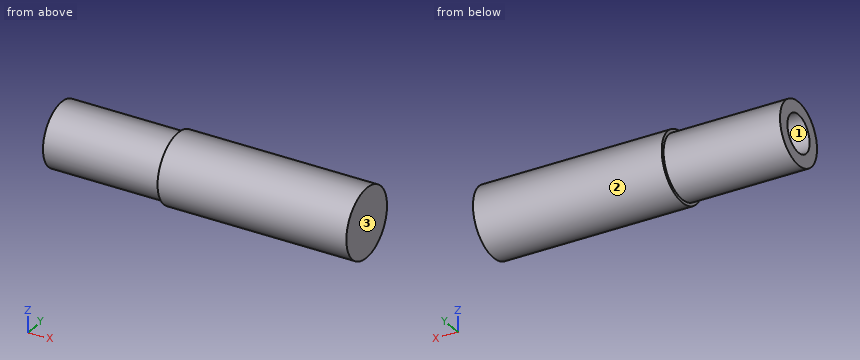
from build123d import *

# Parameters (mm, degrees)
ESQUISSE2_OUTSIDE_W = 23.186
ESQUISSE2_OUTSIDE_H = 23.186
ESQUISSE2_OUTSIDE_R = 5
EXTRUSION1_DEPTH    = 18.5


with BuildPart() as part:
    # Esquisse1 → Révolution1 (revolve)
    with BuildSketch(Plane.XY, mode=Mode.PRIVATE) as r_volution1_sk:
        Polygon((0, 0), (-48.5, 0), (-48.5, -2.5), (-35.5, -2.5), (-35.5, -5.5), (0, -5.5), align=None)
    revolve(r_volution1_sk.sketch.rotate(Axis((-35.5, -5.5, 0), (1, 0, 0)), 180), axis=Axis((-35.5, -5.5, 0), (1, 0, 0)))

    # Esquisse2 outside → Extrusion1 (cut)
    with BuildSketch(Plane.ZY.offset(48.5)):
        with Locations((0, -5.5)):
            Rectangle(ESQUISSE2_OUTSIDE_W, ESQUISSE2_OUTSIDE_H)
        with Locations(Location((0, -5.5, 0), (0, 0, 270))):
            Circle(ESQUISSE2_OUTSIDE_R, mode=Mode.SUBTRACT)
    extrude(amount=-EXTRUSION1_DEPTH, mode=Mode.SUBTRACT)


solid = part.part
Design review of the part built by this model. Coordinates are the model's own, in mm. Face numbers are marked on the shaded views. Give positions to 0.01 mm unless a question says otherwise; leave off trailing zeros. Loops run counter-clockwise (first coordinate to the right, second up) from the corner with the lowest first, then second, coordinate; pieces in that order, holes last. Notation, with made-up numbers: (-3, 18.25) -> (2, 18.25) arc R30 cw to (2, 52.25) -> close; hole circle Ø2 at (46, 86.5). An arc over 180 degrees is marked (long way). One line per question, with ' | ' between items. Start each with the question number.
(1) Insertion check: P1, Ø2, axis at x = -19.5, z = 4, coming from the +Y side; P2, Ø1, axis at x = -35.5, z = 1, coming from the -Y side; P3, Ø2, axis at x = -8.5, z = -1.5, coming from the +Y side. Each pin has a flat end and moves straight along its axis. Give the tip position at first contact, or say it passes through.
(2) We need section C-C (x = -26.5). State the section outline as (y, z) points.
(3) For line 1 (Z direction, x = -43.5, y = -5.5); line 2 (X direction, y = -0.75, z = -2); line 3 (X direction, y = -4.25, z = 0.75), list the stretches that pass through material, from the lowest coordinate up.
(4) Draft analysis for pull direction Z (two halves, no side actions). For the marked faces 1, 2 and 3, state which applies: +Z half, -Z half, draft (parallel to the pull), parting line (faces both ways), or undercut.
(5) We need section D-D (z = 4.5). State the section outline as (x, y) points, and give its area (3 significant figures).
(6) We need section A-A (z = 0). State the section outline as (x, y) points.
(7) We need section B-B (y = -5.5). State the section outline as (x, z) points, and give its area (3 significant figures).
The answers:
1) P1: stops at y = -0.89 | P2: stops at y = -10.47 | P3: stops at y = -0.02
2) outline: circle Ø11 at (-5.5, 0)
3) line 1: z = -5 to -3, 3 to 5 | line 2: x = -30 to 0 | line 3: x = -35.5 to 0
4) face 1: undercut | face 2: parting line | face 3: draft
5) outline: (-48.5, -7.68) -> (-30, -7.68) -> (-30, -8.66) -> (0, -8.66) -> (0, -2.34) -> (-30, -2.34) -> (-30, -3.32) -> (-48.5, -3.32) -> close | area: 270 mm^2
6) outline: (-48.5, -10.5) -> (-30, -10.5) -> (-30, -11) -> (0, -11) -> (0, 0) -> (-30, 0) -> (-30, -0.5) -> (-48.5, -0.5) -> (-48.5, -2.5) -> (-35.5, -2.5) -> (-35.5, -8.5) -> (-48.5, -8.5) -> close
7) outline: (-48.5, -5) -> (-30, -5) -> (-30, -5.5) -> (0, -5.5) -> (0, 5.5) -> (-30, 5.5) -> (-30, 5) -> (-48.5, 5) -> (-48.5, 3) -> (-35.5, 3) -> (-35.5, -3) -> (-48.5, -3) -> close | area: 437 mm^2
